Verification items for the finished model (mm, model axes). Face numbers are marked on the shaded views. A direction names the side the tool comes from. Round coordinates to 2 decimals unless told otherwise and drop trailing zeros. Loops run counter-clockwise (first coordinate to the right, second up) from the corner with the lowest first, then second, coordinate; pieces in that order, holes last. Notation, with made-up numbers: (-24.75, 60.25) -> (16.25, 60.25) arc R27 cw to (16.25, 83.25) -> close; hole circle Ø11 at (4.25, 69.25). An arc over 180 degrees is marked (long way). Write item = value, one per line.
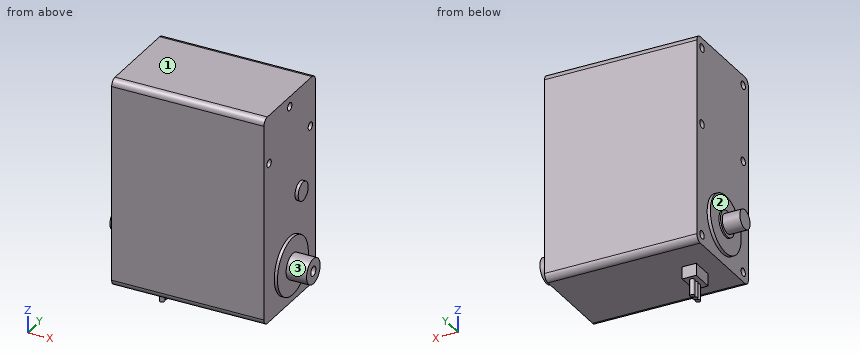
```python
from build123d import *

# Parameters (mm, degrees)
ESQUISSE1_W                         = 47.7
ESQUISSE1_H                         = 65.15
BOSS_EXTRU_1_DEPTH                  = 15
ESQUISSE2_R                         = 9
BOSS_EXTRU_2_DEPTH                  = 1
ESQUISSE3_R                         = 3.95
BOSS_EXTRU_3_DEPTH                  = 6.4
ESQUISSE4_R                         = 4
BOSS_EXTRU_4_DEPTH                  = 0.5
ESQUISSE5_R                         = 3
BOSS_EXTRU_5_DEPTH                  = 5.5
ESQUISSE6_R                         = 2.9
BOSS_EXTRU_6_DEPTH                  = 1
ESQUISSE7_W                         = 4.4
ESQUISSE7_H                         = 6.9
BOSS_EXTRU_7_DEPTH                  = 3.8
ESQUISSE8_R                         = 0.75
BOSS_EXTRU_8_DEPTH                  = 5
DIAM_TRE_DU_PER_AGE_3_0_3_1_D       = 3
DIAM_TRE_DU_PER_AGE_3_0_3_1_DEPTH   = 6.2
DIAM_TRE_DU_PER_AGE_3_0_3_1_TIP     = 0.901290929
DIAM_TRE_DU_PER_AGE_2_5_2_5_1_D     = 2.5
DIAM_TRE_DU_PER_AGE_2_5_2_5_1_DEPTH = 6.2
DIAM_TRE_DU_PER_AGE_2_5_2_5_1_TIP   = 0.751075774
DIAM_TRE_DU_PER_AGE_2_5_2_5_2_D     = 2.5
DIAM_TRE_DU_PER_AGE_2_5_2_5_2_DEPTH = 6.2
DIAM_TRE_DU_PER_AGE_2_5_2_5_2_TIP   = 0.751075774
CONG_1_R                            = 2


with BuildPart() as part:
    # Esquisse1 → Boss.-Extru.1 (new, symmetric)
    with BuildSketch(Plane(origin=(0, 0, 0), x_dir=(1, 0, 0), z_dir=(0, 1, 0))):
        Rectangle(ESQUISSE1_W, ESQUISSE1_H)
    extrude(amount=BOSS_EXTRU_1_DEPTH, both=True)

    # Esquisse2 → Boss.-Extru.2 (add)
    with BuildSketch(Plane(origin=(23.85, 0, 0), x_dir=(0, 0, -1), z_dir=(1, 0, 0))):
        with Locations(Location((20.575, 0, 0), (0, 0, 180))):
            Circle(ESQUISSE2_R)
    boss_extru_2 = extrude(amount=BOSS_EXTRU_2_DEPTH)

    # Sym_trie1: Boss.-Extru.2 across plane
    add(boss_extru_2.mirror(Plane(origin=(0, 0, 0), x_dir=(0, 0, 1), z_dir=(1, 0, 0))))

    # Esquisse3 → Boss.-Extru.3 (add)
    with BuildSketch(Plane(origin=(24.85, 0, 0), x_dir=(0, 0, -1), z_dir=(1, 0, 0))):
        with Locations((20.575, 0)):
            Circle(ESQUISSE3_R)
    extrude(amount=BOSS_EXTRU_3_DEPTH)

    # Esquisse4 → Boss.-Extru.4 (add)
    with BuildSketch(Plane.ZY.offset(24.85)):
        with Locations((-20.575, 0)):
            Circle(ESQUISSE4_R)
    extrude(amount=BOSS_EXTRU_4_DEPTH)

    # Esquisse5 → Boss.-Extru.5 (add)
    with BuildSketch(Plane.ZY.offset(25.35)):
        with Locations((-20.575, 0)):
            Circle(ESQUISSE5_R)
    extrude(amount=BOSS_EXTRU_5_DEPTH)

    # Esquisse6 → Boss.-Extru.6 (add)
    with BuildSketch(Plane(origin=(23.85, 0, 0), x_dir=(0, 0, -1), z_dir=(1, 0, 0))):
        with Locations(Location((-0.075, 6, 0), (0, 0, 180))):
            Circle(ESQUISSE6_R)
    extrude(amount=BOSS_EXTRU_6_DEPTH)

    # Esquisse7 → Boss.-Extru.7 (add)
    with BuildSketch(Plane(origin=(0, 0, -32.575), x_dir=(-1, 0, 0), z_dir=(0, 0, -1))):
        with Locations((15.25, 0)):
            Rectangle(ESQUISSE7_W, ESQUISSE7_H)
    extrude(amount=BOSS_EXTRU_7_DEPTH)

    # Esquisse8 → Boss.-Extru.8 (add)
    with BuildSketch(Plane(origin=(0, 0, -36.375), x_dir=(-1, 0, 0), z_dir=(0, 0, -1))):
        with Locations((15.25, 0)):
            Circle(ESQUISSE8_R)
        with Locations((15.25, -1.6)):
            Circle(ESQUISSE8_R)
        with Locations(Location((15.25, 1.6, 0), (0, 0, 180))):
            Circle(ESQUISSE8_R)
    extrude(amount=BOSS_EXTRU_8_DEPTH)

    # Diam_tre du per_age _3.0 _3_1
    with Locations(Plane(origin=(31.25, 0, 0), x_dir=(0, 0, -1), z_dir=(1, 0, 0))):
        with Locations((20.575, 0)):
            Hole(DIAM_TRE_DU_PER_AGE_3_0_3_1_D / 2, depth=DIAM_TRE_DU_PER_AGE_3_0_3_1_DEPTH)
            with Locations((0, 0, -(DIAM_TRE_DU_PER_AGE_3_0_3_1_DEPTH + DIAM_TRE_DU_PER_AGE_3_0_3_1_TIP / 2))):  # 118° drill point
                Cone(0, DIAM_TRE_DU_PER_AGE_3_0_3_1_D / 2, DIAM_TRE_DU_PER_AGE_3_0_3_1_TIP, mode=Mode.SUBTRACT)

    # Diam_tre du per_age _2.5 _2.5_1
    with Locations(Plane(origin=(23.85, 0, 0), x_dir=(0, 0, -1), z_dir=(1, 0, 0))):
        with Locations((-29.425, 0), (-17.425, 12), (-17.425, -12)):
            Hole(DIAM_TRE_DU_PER_AGE_2_5_2_5_1_D / 2, depth=DIAM_TRE_DU_PER_AGE_2_5_2_5_1_DEPTH)
            with Locations((0, 0, -(DIAM_TRE_DU_PER_AGE_2_5_2_5_1_DEPTH + DIAM_TRE_DU_PER_AGE_2_5_2_5_1_TIP / 2))):  # 118° drill point
                Cone(0, DIAM_TRE_DU_PER_AGE_2_5_2_5_1_D / 2, DIAM_TRE_DU_PER_AGE_2_5_2_5_1_TIP, mode=Mode.SUBTRACT)

    # Diam_tre du per_age _2.5 _2.5_2
    with Locations(Plane.ZY.offset(23.85)):
        with Locations((29.5, 12), (-29.5, 12), (29.5, -12), (-29.5, -12), (5.5, 12), (5.5, -12)):
            Hole(DIAM_TRE_DU_PER_AGE_2_5_2_5_2_D / 2, depth=DIAM_TRE_DU_PER_AGE_2_5_2_5_2_DEPTH)
            with Locations((0, 0, -(DIAM_TRE_DU_PER_AGE_2_5_2_5_2_DEPTH + DIAM_TRE_DU_PER_AGE_2_5_2_5_2_TIP / 2))):  # 118° drill point
                Cone(0, DIAM_TRE_DU_PER_AGE_2_5_2_5_2_D / 2, DIAM_TRE_DU_PER_AGE_2_5_2_5_2_TIP, mode=Mode.SUBTRACT)

    # Cong_1
    cong_1_edges = [part.edges().sort_by_distance(p)[0] for p in [
        (0, 15, -32.575),
        (0, -15, -32.575),
        (0, -15, 32.575),
        (0, 15, 32.575),
    ]]
    fillet(cong_1_edges, radius=CONG_1_R)


solid = part.part
```
(1) Sectioned sample at C-C, the plane y = -5. Record the cut outline in (x, z) (3 decimals), and give its area (3 significant figures).
Filled sheet:
outline = (-24.85, -28.058) -> (-23.85, -28.058) -> (-23.85, -32.575) -> (23.85, -32.575) -> (23.85, -28.058) -> (24.85, -28.058) -> (24.85, -13.092) -> (23.85, -13.092) -> (23.85, 32.575) -> (-23.85, 32.575) -> (-23.85, -13.092) -> (-24.85, -13.092) -> close
area = 3,140 mm2
(2) Sectioned sample at A-A, the plane x = 20. Record the cut outline in (y, z) (3 decimals).
Filled sheet:
outline = (-15, -30.575) arc R2 ccw to (-13, -32.575) -> (13, -32.575) arc R2 ccw to (15, -30.575) -> (15, 30.575) arc R2 ccw to (13, 32.575) -> (-13, 32.575) arc R2 ccw to (-15, 30.575) -> close; hole circle Ø2.5 at (-12, 17.425); hole circle Ø2.5 at (0, 29.425); hole circle Ø2.5 at (12, 17.425)
(3) Sectioned sample at B-B, the plane x = 7.5. Record the cut outline in (y, z) (3 decimals).
Filled sheet:
outline = (-15, -30.575) arc R2 ccw to (-13, -32.575) -> (13, -32.575) arc R2 ccw to (15, -30.575) -> (15, 30.575) arc R2 ccw to (13, 32.575) -> (-13, 32.575) arc R2 ccw to (-15, 30.575) -> close
(4) Go/stop test with flat-tipped pins: pin 1 Ø4 at (y, z) = (-9.5, -6.5) entering from -X; pin 2 Ø12 at (x, y) = (-23, 5) entering from -Z (3 decimals); pin 3 Ø9 at (y, z) = (7, -13.5) entering from -X. Record where each tip stops, or that it passes through.
Filled sheet:
pin_1 = -23.85
pin_2 = -36.375
pin_3 = -24.85
(5) Material ranges on probe 1 along Z at (x, y) = (-20.75, 12) (3 decimals); probe 2 along Y at (x, z) = (-21.5, 5.5); probe 3 along Y at (x, z) = (-20, 29), recorded low to high. Write a range as from..to.
Filled sheet:
probe_1 = -32.575..-30.75, -28.25..4.25, 6.75..28.25, 30.75..32.575
probe_2 = -15..-13.25, -10.75..10.75, 13.25..15
probe_3 = -15..-13.15, -10.85..10.85, 13.15..15
(6) Set-up check for the marked faces 1, 2 and 3: record each of +Z, -Z, +X, -X, +Y, -Y from which the full face is reachable in a straight line by a thin tool's end or side.
Filled sheet:
face_1 = +Z, +X, -X, +Y, -Y
face_2 = -X
face_3 = +X
(7) Sectioned sample at D-D, the plane z = -13.5. Record the cut outline in (x, y), and give its area (3 significant figures).
Filled sheet:
outline = (-24.85, -5.56) -> (-23.85, -5.56) -> (-23.85, -15) -> (23.85, -15) -> (23.85, -5.56) -> (24.85, -5.56) -> (24.85, 5.56) -> (23.85, 5.56) -> (23.85, 15) -> (-23.85, 15) -> (-23.85, 5.56) -> (-24.85, 5.56) -> close
area = 1,450 mm2
